The listing builds one solid part. Answer for the finished solid, in the listing's coordinates (mm). A direction names the side the tool comes from. Give positions to 0.01 mm unless a question says otherwise; leave off trailing zeros. Loops run counter-clockwise (first coordinate to the right, second up) from the corner with the lowest first, then second, coordinate; pieces in that order, holes last. Notation, with made-up numbers: (3.25, 66) - (15.25, 66) arc R35 cw to (15.25, 99) - close; hole circle Ø6 at (68, 18). An arc over 180 degrees is marked (long way). Write item = value, one per line. Start each with the question number.
1) The mould has two halves that part along Z. Classify faces 5 (the flat face through (4, 0, 6)), 6 (the cylindrical face through (9.82, 0.1, -2.55)), 7 (the cylindrical face through (-6.124, 6.144, 0.084)): +Z half, -Z half, draft (parallel to the pull), parting line (faces both ways), or undercut.
2) Flat-ended cylindrical pins translate along their axes: P1, Ø0.8, axis at y = -2.5, z = -0.5, coming from the +X side; P2, Ø1.1, axis at y = 2.5, z = -0.5, coming from the +X side; P3, Ø6, axis at y = 0, z = 0.5, coming from the +X side. Find the tip coordinate at first contact, or state that the pin passes through.
3) The part is cut by section D-D on y = 3.5. State how many separate pieces and enclosed holes the cut face has, plus the area to 3 significant figures.
4) The part is cut by section B-B on y = 0. Write down the section's boundary in (x, z).
5) Which of the six approach directions +Z, -Z, +X, -X, +Y, -Y give full straight-line access (tool end or side, diameter ignored) to faces 1 (the flat face through (-1.87, -3.04, 0.08)), 2 (the flat face through (6.5, 0, 1)), 3 (the flat face through (10, -5.25, 0)), 4 (the cylindrical face through (-6.144, -6.124, 0.084))?
6) Consider probe 1 along Y at (x, z) = (4.75, 0); probe 2 along X at (y, z) = (-3.5, 5); probe 3 along Y at (x, z) = (-2, -2). Determine where each line is inside the solid, lowest interval first.
7) The part is cut by section C-C on x = 8. Write down the section's boundary in (y, z).
8) The part is cut by section A-A on x = 4.5. Write down the section's boundary in (y, z), plus the area to 3 significant figures.
from build123d import *

# Parameters (mm, degrees)
F1_DEPTH = 6
F3_DEPTH = 10
F5_DEPTH = 8
F6_R     = 1.27


with BuildPart() as f1:
    # F0 (on Top) → F1 (new body, symmetric)
    with BuildSketch(Plane.XY):
        with BuildLine():
            Line((6.5, -5.25), (6.5, 5.25))
            ThreePointArc((6.5, 5.25), (6.133883, 6.133883), (5.25, 6.5))
            Line((5.25, 6.5), (-5.25, 6.5))
            ThreePointArc((-5.25, 6.5), (-6.133883, 6.133883), (-6.5, 5.25))
            Line((-6.5, 5.25), (-6.5, -5.25))
            ThreePointArc((-6.5, -5.25), (-6.133883, -6.133883), (-5.25, -6.5))
            Line((-5.25, -6.5), (5.25, -6.5))
            ThreePointArc((5.25, -6.5), (6.133883, -6.133883), (6.5, -5.25))
        make_face()
    extrude(amount=F1_DEPTH, both=True)

    # F2 (on Top) → F3 (cut, symmetric)
    with BuildSketch(Plane.XY):
        with BuildLine():
            ThreePointArc((0.889914, -2.1566), (0.928239, -2.163918), (0.961171, -2.184843))
            Line((0.961171, -2.184843), (2.745753, -3.863205))
            Line((2.745753, -3.863205), (1.752595, -3.863205))
            ThreePointArc((1.752595, -3.863205), (1.466924, -3.981534), (1.348595, -4.267205))
            Line((1.348595, -4.267205), (1.348595, -4.749805))
            ThreePointArc((1.348595, -4.749805), (1.466924, -5.035476), (1.752595, -5.153805))
            Line((1.752595, -5.153805), (4.749795, -5.153805))
            ThreePointArc((4.749795, -5.153805), (5.035466, -5.035476), (5.153795, -4.749805))
            Line((5.153795, -4.749805), (5.153795, -1.752605))
            ThreePointArc((5.153795, -1.752605), (5.035471, -1.466932), (4.749802, -1.348599))
            Line((4.749802, -1.348599), (4.267202, -1.348599))
            ThreePointArc((4.267202, -1.348599), (3.981531, -1.466927), (3.863202, -1.752599))
            Line((3.863202, -1.752599), (3.863202, -2.745756))
            Line((3.863202, -2.745756), (2.184831, -0.961164))
            ThreePointArc((2.184831, -0.961164), (2.163912, -0.928237), (2.156595, -0.889919))
            Line((2.156595, -0.889919), (2.156595, 0.889909))
            ThreePointArc((2.156595, 0.889909), (2.163912, 0.928229), (2.184834, 0.961157))
            Line((2.184834, 0.961157), (3.863202, 2.745746))
            Line((3.863202, 2.745746), (3.863202, 1.752589))
            ThreePointArc((3.863202, 1.752589), (3.981531, 1.466917), (4.267202, 1.348589))
            Line((4.267202, 1.348589), (4.749802, 1.348589))
            ThreePointArc((4.749802, 1.348589), (5.035473, 1.466917), (5.153802, 1.752589))
            Line((5.153802, 1.752589), (5.153802, 4.749789))
            ThreePointArc((5.153802, 4.749789), (5.035477, 5.035475), (4.749794, 5.153807))
            Line((4.749794, 5.153807), (1.752594, 5.153807))
            ThreePointArc((1.752594, 5.153807), (1.466922, 5.035478), (1.348594, 4.749807))
            Line((1.348594, 4.749807), (1.348594, 4.267207))
            ThreePointArc((1.348594, 4.267207), (1.466922, 3.981536), (1.752594, 3.863207))
            Line((1.752594, 3.863207), (2.745751, 3.863207))
            Line((2.745751, 3.863207), (0.961159, 2.184836))
            ThreePointArc((0.961159, 2.184836), (0.928232, 2.163916), (0.889914, 2.1566))
            Line((0.889914, 2.1566), (-0.889914, 2.1566))
            ThreePointArc((-0.889914, 2.1566), (-0.928238, 2.163918), (-0.961169, 2.184841))
            Line((-0.961169, 2.184841), (-2.745757, 3.863209))
            Line((-2.745757, 3.863209), (-1.7526, 3.863209))
            ThreePointArc((-1.7526, 3.863209), (-1.466929, 3.981538), (-1.3486, 4.267209))
            Line((-1.3486, 4.267209), (-1.3486, 4.749809))
            ThreePointArc((-1.3486, 4.749809), (-1.466937, 5.035473), (-1.752607, 5.153794))
            Line((-1.752607, 5.153794), (-4.749807, 5.153794))
            ThreePointArc((-4.749807, 5.153794), (-5.035478, 5.035465), (-5.153807, 4.749794))
            Line((-5.153807, 4.749794), (-5.153807, 1.752594))
            ThreePointArc((-5.153807, 1.752594), (-5.035478, 1.466922), (-4.749807, 1.348594))
            Line((-4.749807, 1.348594), (-4.267207, 1.348594))
            ThreePointArc((-4.267207, 1.348594), (-3.981536, 1.466922), (-3.863207, 1.752594))
            Line((-3.863207, 1.752594), (-3.863207, 2.745751))
            Line((-3.863207, 2.745751), (-2.184836, 0.961159))
            ThreePointArc((-2.184836, 0.961159), (-2.163916, 0.928232), (-2.1566, 0.889914))
            Line((-2.1566, 0.889914), (-2.1566, -0.889914))
            ThreePointArc((-2.1566, -0.889914), (-2.163918, -0.928238), (-2.184841, -0.961169))
            Line((-2.184841, -0.961169), (-3.863209, -2.745757))
            Line((-3.863209, -2.745757), (-3.863209, -1.7526))
            ThreePointArc((-3.863209, -1.7526), (-3.981538, -1.466929), (-4.267209, -1.3486))
            Line((-4.267209, -1.3486), (-4.749809, -1.3486))
            ThreePointArc((-4.749809, -1.3486), (-5.035481, -1.466929), (-5.153809, -1.7526))
            Line((-5.153809, -1.7526), (-5.153809, -4.7498))
            ThreePointArc((-5.153809, -4.7498), (-5.035481, -5.035471), (-4.749809, -5.1538))
            Line((-4.749809, -5.1538), (-1.752609, -5.1538))
            ThreePointArc((-1.752609, -5.1538), (-1.466938, -5.035471), (-1.348609, -4.7498))
            Line((-1.348609, -4.7498), (-1.348609, -4.2672))
            ThreePointArc((-1.348609, -4.2672), (-1.466935, -3.981539), (-1.752594, -3.863207))
            Line((-1.752594, -3.863207), (-2.745751, -3.863207))
            Line((-2.745751, -3.863207), (-0.961159, -2.184836))
            ThreePointArc((-0.961159, -2.184836), (-0.928232, -2.163916), (-0.889914, -2.1566))
            Line((-0.889914, -2.1566), (0.889914, -2.1566))
        make_face()
    extrude(amount=F3_DEPTH, both=True, mode=Mode.SUBTRACT)

    # F4 (on face) → F5 (join)
    with BuildSketch(Plane.YZ.offset(6.5)):
        with BuildLine():
            ThreePointArc((1, 2.345741), (0, -2.55), (-1, 2.345741))
            Line((-1, 2.345741), (-1, 6))
            Line((-1, 6), (-5.25, 6))
            Line((-5.25, 6), (-5.25, -6))
            Line((-5.25, -6), (5.25, -6))
            Line((5.25, -6), (5.25, 6))
            Line((5.25, 6), (1, 6))
            Line((1, 6), (1, 2.345741))
        make_face()
    extrude(amount=F5_DEPTH)

    # F6
    f6_edges = [f1.edges().sort_by_distance(p)[0] for p in [
        (14.5, 0, -2.55),
    ]]
    fillet(f6_edges, radius=F6_R)


solid = f1.part
Answer below:
q1.face_5 = +Z half
q1.face_6 = undercut
q1.face_7 = draft
q2.P1 = 14.15
q2.P2 = 14.28
q2.P3 = 14.45
q3.separate_pieces = 3
q3.enclosed_holes = 0
q3.area = 185 mm2
q4.outline = (-6.5, -6) - (-2.16, -6) - (-2.16, 6) - (-6.5, 6) - close; (2.16, -6) - (14.5, -6) - (14.5, -3.82) arc R1.27 ccw to (13.23, -2.55) - (6.5, -2.55) - (6.5, 6) - (2.16, 6) - close
q5.face_1 = +Z, -Z
q5.face_2 = +X
q5.face_3 = +Z, -Z, +X, -Y
q5.face_4 = +Z, -Z, -X, -Y
q6.probe_1 = -6.5 to -5.15, -1.35 to 1.35, 5.15 to 6.5
q6.probe_2 = -6.5 to -5.15, -2.36 to 2.36, 5.15 to 14.5
q6.probe_3 = -6.5 to -5.15, -3.86 to -3.16, 3.16 to 3.86, 5.15 to 6.5
q7.outline = (-5.25, -6) - (5.25, -6) - (5.25, 6) - (1, 6) - (1, 2.35) arc R2.55 cw (long way) to (-1, 2.35) - (-1, 6) - (-5.25, 6) - close
q8.outline = (-6.5, -6) - (-5.15, -6) - (-5.15, 6) - (-6.5, 6) - close; (-1.35, -6) - (1.35, -6) - (1.35, 6) - (-1.35, 6) - close; (5.15, -6) - (6.5, -6) - (6.5, 6) - (5.15, 6) - close
q8.area = 64.7 mm2
